Input: part model. Units: mm. Frame: model coordinates. A direction names the side the tool comes from. Round coordinates to 2 decimals unless told otherwise and drop trailing zeros. Loops run counter-clockwise (first coordinate to the right, second up) from the corner with the lowest first, then second, coordinate; pieces in that order, holes last. Notation, with made-up numbers: M 33.25,33 L 52.25,33 A5 cw 52.25,41 Z; hole C 46,52.25 d4. An arc over 180 degrees is marked long. Put each result on its own line as item: value. Start each with the question number.
1) Reachability of faces 1 (the face through (-22, 0, 49)), 2 (the face through (0, 0, -4)) from +Z, -Z, +X, -X, +Y, -Y: full face, straight path, thin tool, end or side. Return the list, or none.
2) Pin query (flat end, axial travel): pin 1 (10 mm diameter, centred on x = 8.5, z = 42, fed in from +Y); pin 2 (2 mm diameter, centred on x = 10.5, y = 3.5, fed in from +Z); pin 3 (3.5 mm diameter, centred on x = 0, y = -22, fed in from -Z). Return the tip coordinate at first contact, or that it passes through.
3) Section A-A on x = 0. Output: boundary loops of the cut face in (y, z).
4) Draft query along X for faces 3 (the face through (-23.6, -1.2, 51.5)), 4 (the face through (-0.867, -3.905, -1.972)), 5 (the face through (0, 0, 80.5)), 6 (the face through (22, 0, 49)). Return one class per face: +X half, -X half, draft (parallel to the pull), parting line (faces both ways), or undercut.
5) Section B-B on z = 20.5. Output: boundary loops of the cut face in (x, y), plus the area to 3 significant figures.
6) Line query: probe 1 along Y at (x, z) = (0, 50); probe 2 along Y at (x, z) = (0, 52.4); probe 3 along X at (y, z) = (0, 52). Output: solid intervals per line, ascending.
Autodesk Inventor part; units mm, degrees
ref_plane "Work Plane1" through (0, 0, 54) normal (0, 0, 1) x (1, 0, 0)
ref_plane "YZ Plane" through (0, 0, 0) normal (1, 0, 0) x (0, 1, 0)
ref_plane "XZ Plane" through (0, 0, 0) normal (0, 1, 0) x (-1, 0, 0)
sketch "Sketch1" plane through (0, 0, 0) normal (0, 0, 1) x (1, 0, 0)
  circle A0 centre (0, 0) radius 30
  dimension "d0" = 60
extrude "Extrusion1" add sketch "Sketch1" along normal blind 41
ref_plane "Work Plane1" through (0, 0, 54) normal (0, 0, 1) x (1, 0, 0)
sketch "Sketch2" plane through (0, 0, 54) normal (0, 0, 1) x (1, 0, 0)
  circle A0 centre (0, 0) radius 26
  dimension "d4" = 52
loft "Loft1" add profiles "Sketch2" section 1 edges at (-30, 0, 41)
sketch "Sketch4" plane through (0, 0, 54) normal (0, 0, 1) x (1, 0, 0)
  point P0 (0, 0)
sketch "Sketch5" plane through (0, 0, 54) normal (0, 0, 1) x (1, 0, 0)
  circle A0 centre (0, 22) radius 2
  circle A1 centre (0, -22) radius 2
  circle A2 centre (0, 0) radius 22
  circle A3 centre (-22, 0) radius 2
  circle A4 centre (22, 0) radius 2
  dimension "d11" = 4
  dimension "d12" = 44
extrude "Extrusion2" cut sketch "Sketch5" against normal blind 5 contours A0 A2 | A2 A0 | A3 A2 | A2 A3 | A4 A2 | A2 A4 | A2 A1 | A1 A2
sketch "Sketch6" plane through (0, 0, 0) normal (0, 0, -1) x (-1, 0, 0)
  point P0 (0, 0)
sketch "Sketch7" plane through (0, 0, 54) normal (0, 0, 1) x (1, 0, 0)
  circle A0 centre (0, 0) radius 4
  dimension "d16" = 8
extrude "Extrusion3" add sketch "Sketch7" along normal blind 26.5 and the other way blind 58
properties part number "CH-1-02-driveMotor"
Geometry results:
1. face 1: +Z
1. face 2: -Z, +X, -X, +Y, -Y
2. pin 1: stops at y = 29.78
2. pin 2: stops at z = 54
2. pin 3: stops at z = 0
3. outline: M -30,0 L -4,0 L -4,-4 L 4,-4 L 4,0 L 30,0 L 30,41 L 26,54 L 24,54 L 24,49 L 20,49 L 20,54 L 4,54 L 4,80.5 L -4,80.5 L -4,54 L -20,54 L -20,49 L -24,49 L -24,54 L -26,54 L -30,41 Z
4. face 3: undercut
4. face 4: parting line
4. face 5: draft
4. face 6: undercut
5. outline: C 0,0 d60
5. area: 2,830 mm²
6. probe 1: y = -27.23 to -24, -20 to 20, 24 to 27.23
6. probe 2: y = -26.49 to -24, -20 to 20, 24 to 26.49
6. probe 3: x = -26.62 to -24, -20 to 20, 24 to 26.62
